Geometry: final body of the model. Coordinates: model frame, mm. A direction names the side the tool comes from. Coordinates: 2 decimals unless noted, no trailing zeros. Write each loop counter-clockwise with the first axis right and the second up, starting at its lowest first coordinate (ties: lowest second). Pieces come first, ordered by that corner, then holes.
from build123d import *

# Parameters (mm, degrees)
CROQUIS1_W              = 700
CROQUIS1_H              = 345
SALIENTE_EXTRUIR1_DEPTH = 38.1
CROQUIS2_W              = 370
CROQUIS2_H              = 265
CORTAR_EXTRUIR1_DEPTH   = 38.1
REDONDEO1_R             = 15
CROQUIS3_R              = 115
SALIENTE_EXTRUIR2_DEPTH = 70
CROQUIS4_R              = 45
CORTAR_EXTRUIR2_DEPTH   = 70
CROQUIS5_W              = 63
CROQUIS5_H              = 247.074165674
CORTAR_EXTRUIR3_DEPTH   = 26


with BuildPart() as part:
    # Croquis1 → Saliente-Extruir1 (new body)
    with BuildSketch(Plane(origin=(0, 0, 0), x_dir=(1, 0, 0), z_dir=(0, 1, 0))):
        Rectangle(CROQUIS1_W, CROQUIS1_H)
    extrude(amount=SALIENTE_EXTRUIR1_DEPTH)

    # Croquis2 → Cortar-Extruir1 (cut)
    with BuildSketch(Plane(origin=(0, 38.1, 0), x_dir=(1, 0, 0), z_dir=(0, 1, 0))):
        with Locations((-125, 0)):
            Rectangle(CROQUIS2_W, CROQUIS2_H)
    extrude(amount=-CORTAR_EXTRUIR1_DEPTH, mode=Mode.SUBTRACT)

    # Redondeo1
    redondeo1_edges = [part.edges().sort_by_distance(p)[0] for p in [
        (-310, 19.05, 132.5),
        (-310, 19.05, -132.5),
        (60, 19.05, -132.5),
        (60, 19.05, 132.5),
    ]]
    fillet(redondeo1_edges, radius=REDONDEO1_R)

    # Croquis3 → Saliente-Extruir2 (add)
    with BuildSketch(Plane(origin=(0, 38.1, 0), x_dir=(1, 0, 0), z_dir=(0, 1, 0))):
        with Locations((235, 0)):
            Circle(CROQUIS3_R)
    extrude(amount=SALIENTE_EXTRUIR2_DEPTH)

    # Croquis4 → Cortar-Extruir2 (cut)
    with BuildSketch(Plane(origin=(0, 108.1, 0), x_dir=(1, 0, 0), z_dir=(0, 1, 0))):
        with Locations(Location((235, 0, 0), (0, 0, 270))):
            Circle(CROQUIS4_R)
    extrude(amount=-CORTAR_EXTRUIR2_DEPTH, mode=Mode.SUBTRACT)

    # Croquis5 → Cortar-Extruir3 (cut)
    with BuildSketch(Plane(origin=(0, 108.1, 0), x_dir=(1, 0, 0), z_dir=(0, 1, 0))):
        with Locations((235, 0)):
            Rectangle(CROQUIS5_W, CROQUIS5_H)
    extrude(amount=-CORTAR_EXTRUIR3_DEPTH, mode=Mode.SUBTRACT)


solid = part.part
Item 1: Section A-A, the plane x = -255. Output: boundary loops of the cut face in (y, z), plus the area to 3 significant figures.
Derived:
outline: (0, -172.5) - (38.1, -172.5) - (38.1, -132.5) - (0, -132.5) - close; (0, 132.5) - (38.1, 132.5) - (38.1, 172.5) - (0, 172.5) - close
area: 3,050 mm2
Item 2: Set-up query: faces 4 (the cylindrical face through (-305.49, 18.78, 128.22)), 5 (the flat face through (203.5, 95, -71)), 6 (the flat face through (350, 19, 2)), 7 (the cylindrical face through (248.52, 65.81, 42.92)). Return all of +Z, -Z, +X, -X, +Y, -Y with unobstructed straight access to the full face (end or side cutting, diameter ignored); none if empty.
Derived:
face 4: +Y, -Y
face 5: +Z, -Z, +Y
face 6: +Z, -Z, +X, +Y, -Y
face 7: +Y
Item 3: Section B-B, the plane z = -13. Output: boundary loops of the cut face in (x, y), plus the area to 3 significant figures.
Derived:
outline: (-350, 0) - (-310, 0) - (-310, 38.1) - (-350, 38.1) - close; (60, 0) - (350, 0) - (350, 38.1) - (349.26, 38.1) - (349.26, 108.1) - (278.08, 108.1) - (278.08, 38.1) - (191.92, 38.1) - (191.92, 108.1) - (120.74, 108.1) - (120.74, 38.1) - (60, 38.1) - close
area: 22,500 mm2
Item 4: Pull-direction query (Z, two-part tool) for faces 1 (the flat face through (266.5, 95, -71)), 2 (the flat face through (236, 38.1, -1)), 3 (the flat face through (-5, 19, -172.5)); classes: released by +Z, released by -Z, zero draft, split by the parting line, or undercut.
Derived:
face 1: zero draft
face 2: undercut
face 3: released by -Z
Item 5: Pin query (flat end, axial travel): pin 1 (21 mm diameter, centred on y = 98.5, z = 60, fed in from +X); pin 2 (21 mm diameter, centred on y = 89, z = -73.5, fed in from -X); pin 3 (13 mm diameter, centred on y = 98, z = -78.5, fed in from +X). Return the tip coordinate at first contact, or that it passes through.
Derived:
pin 1: stops at x = 338.8
pin 2: stops at x = 138.79
pin 3: stops at x = 324.67
Item 6: Section C-C, the plane y = 18.5. Output: boundary loops of the cut face in (x, z).
Derived:
outline: (-350, -172.5) - (350, -172.5) - (350, 172.5) - (-350, 172.5) - close; hole (-310, -117.5) arc R15 ccw to (-295, -132.5) - (45, -132.5) arc R15 ccw to (60, -117.5) - (60, 117.5) arc R15 ccw to (45, 132.5) - (-295, 132.5) arc R15 ccw to (-310, 117.5) - close
Item 7: Material intervals for probe 1 along X at (y, z) = (36, -86); probe 2 along Z at (x, y) = (235, 61.5); probe 3 along Z at (x, y) = (-204, 18.5), sorted ascending.
Derived:
probe 1: x = -350 to -310, 60 to 350
probe 2: z = -115 to -45, 45 to 115
probe 3: z = -172.5 to -132.5, 132.5 to 172.5
Item 8: Section D-D, the plane x = 235. Output: boundary loops of the cut face in (y, z), plus the area to 3 significant figures.
Derived:
outline: (0, -172.5) - (38.1, -172.5) - (38.1, -115) - (82.1, -115) - (82.1, -45) - (38.1, -45) - (38.1, 45) - (82.1, 45) - (82.1, 115) - (38.1, 115) - (38.1, 172.5) - (0, 172.5) - close
area: 19,300 mm2
